```python
from build123d import *

# Parameters (mm, degrees)
F0_R          = 4.7625
F0_R_2        = 2.15265
F1_DEPTH      = 138.557
F3_R          = 2.15265
F4_DEPTH      = 3.2512
F4_DEPTH_BACK = 148.3106
F5_DEPTH      = 138.557
F7_R          = 6.35
F7_R_2        = 2.15265
F8_DEPTH      = 25.4


with BuildPart() as f1:
    # F0 (on Top) → F1 (new body)
    with BuildSketch(Plane.XY):
        Circle(F0_R)
        Circle(F0_R_2, mode=Mode.SUBTRACT)
    extrude(amount=F1_DEPTH)

    # F3 (on face) → F4 (join, two sides)
    with BuildSketch(Plane.XY.offset(138.557)) as f4_sk:
        Polygon((4.7625, 0), (2.38125, 4.1244459855), (-2.38125, 4.1244459855), (-4.7625, 0), (-2.38125, -4.1244459855), (2.38125, -4.1244459855), align=None)
        Circle(F3_R, mode=Mode.SUBTRACT)
    extrude(amount=F4_DEPTH)
    extrude(f4_sk.sketch, amount=-F4_DEPTH_BACK)

    # F5 (cut, through all): a face of the model
    f5_faces = [f1.faces().sort_by_distance(p)[0] for p in [
        (-3.7942237484, 2.1905961025, 138.557),
    ]]
    extrude(f5_faces, amount=-F5_DEPTH, mode=Mode.SUBTRACT)

    # F7 (on offset) → F8 (join)
    with BuildSketch(Plane.XY.offset(91.8845)):
        Circle(F7_R)
        Circle(F7_R_2, mode=Mode.SUBTRACT)
    extrude(amount=-F8_DEPTH)


solid = f1.part
```
The model under review builds one solid part; all positions refer to its coordinate system, in mm. A direction names the side the tool comes from. Round coordinates to 2 decimals unless told otherwise and drop trailing zeros. Order: outer loops, then holes, each group sorted by start corner. A loop starts at its lowest first (then second) coordinate and runs counter-clockwise, first axis right, second up.
Item 1: Add section B-B, the plane z = 9. State the section outline as (x, y) points (1 decimal), and give its area (3 significant figures).
Working result:
outline: (-4.8, 0) arc R4.8 ccw (long way) to (-2.4, 4.1) - close; hole circle Ø4.3 at (0, 0)
area: 54.6 mm2
Item 2: Machinability: for faces 1 (the flat face through (0, -4.124, 140)), 2 (the flat face through (-3.59, -2.03, 140.16)), 3 (the flat face through (0, 4.124, -5)), 4 (the flat face through (4, -2, 0)), 5 (the flat face through (4, 2, 138.557)), which of the approach directions +Z, -Z, +X, -X, +Y, -Y give a long, thin tool a straight path to every point of the face, cutting with its end or side? Answer none if there is none.
Working result:
face 1: +Z, +X, -X, -Y
face 2: +Z, -X, -Y
face 3: -Z, +X, -X, +Y
face 4: -Z, +X, -Y
face 5: +Z, +X, +Y
Item 3: Add section A-A, the plane x = 0. State the section outline as (y, z) points, and give its area (3 significant figures).
Working result:
outline: (-6.35, 66.48) - (-4.76, 66.48) - (-4.76, 0) - (-4.12, 0) - (-4.12, -9.75) - (-2.15, -9.75) - (-2.15, 141.81) - (-4.12, 141.81) - (-4.12, 138.56) - (-4.76, 138.56) - (-4.76, 91.88) - (-6.35, 91.88) - close; (2.15, -9.75) - (4.12, -9.75) - (4.12, 0) - (4.76, 0) - (4.76, 66.48) - (6.35, 66.48) - (6.35, 91.88) - (4.76, 91.88) - (4.76, 138.56) - (4.12, 138.56) - (4.12, 141.81) - (2.15, 141.81) - close
area: 855 mm2
Item 4: For pin 1 (6 mm diameter, centred on y = -3, z = 125, fed in from -X); pin 2 (2 mm diameter, centred on y = -4.5, z = 18.5, fed in from +X); pin 3 (3 mm diameter, centred on x = 1.5, z = 39.5, fed in from -Y), all flat-tipped, find the tip position at first contact; note any pin that passes through.
Working result:
pin 1: stops at x = -4.76
pin 2: stops at x = 3.23
pin 3: stops at y = -4.76
Item 5: Add section C-C, the plane z = 88. State the section outline as (x, y) points.
Working result:
outline: circle Ø12.7 at (0, 0); hole circle Ø4.31 at (0, 0)
Item 6: To check wall thickness, follow probe 1 along Y at (x, z) = (0, 16.5); probe 2 along Y at (x, z) = (0, 140.45); probe 3 along Z at (x, y) = (5.5, -0.5). State the ranges of each line that lie inside material, in increasing order.
Working result:
probe 1: y = -4.76 to -2.15, 2.15 to 4.76
probe 2: y = -4.12 to -2.15, 2.15 to 4.12
probe 3: z = 66.48 to 91.88
